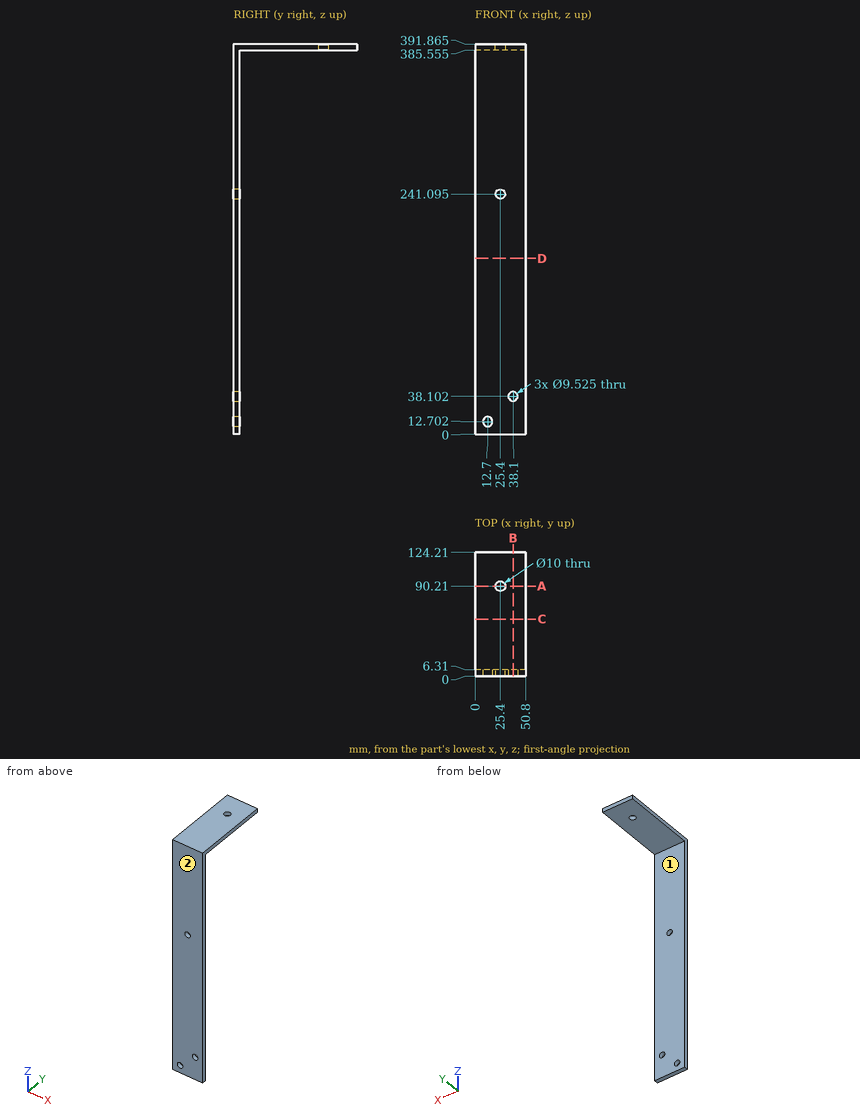
Could you check a few things on this drawing? It's one solid part, dimensions in mm from its lowest x, y, z. A direction names the side the tool comes from. Coordinates: 2 decimals unless noted, no trailing zeros. Write each loop counter-clockwise with the first axis right and the second up, starting at its lowest first coordinate (ties: lowest second). Pieces come first, ordered by that corner, then holes. Notation, with made-up numbers: M 27.25,-25.5 L 41.25,-25.5 A18 ccw 41.25,-18.5 Z; hole C 88,43.5 d4. An arc over 180 degrees is marked long. Answer as CSV lines item,"result". Start each with the question number.
Q1. Suppose I cut it at D-D, the plane z = 176.5. List the corners of the cut face in (x, y) for me, then the cut area to 3 significant figures.
Q2. For the marked faces 1 and 2, which set-ups out of +Z, -Z, +X, -X, +Y, -Y let a thin tool reach every point of the face, with its end or its side?
Q3. Suppose I cut it at A-A, the plane y = 90.21. List the corners of the cut face in (x, z) for me (3 decimals).
Q4. Suppose I cut it at B-B, the plane x = 38.1. List the corners of the cut face in (y, z) for me (1 decimal).
Q5. Suppose I cut it at C-C, the plane y = 57. List the corners of the cut face in (x, z) for me (3 decimals).
Q6. I need wall thicknesses on probe 1 along Z at (x, y) = (38.1, 2) (1 decimal); probe 2 along Z at (x, y) = (12.7, 3) (1 decimal); probe 3 along Z at (x, y) = (36, 72) (3 decimals). Which ranges of each line are inside material? Lowest first, please. Write a range as [from, to].
Q7. Will these pins go through, and if not, where does the flat tip stop? pin 1 Ø12 at (x, z) = (29, 93) entering from +Y; pin 2 Ø15 at (x, y) = (18.5, 56) entering from -Z (3 decimals).
Entries:
1,outline,"M 0,0 L 50.8,0 L 50.8,6.31 L 0,6.31 Z"
1,area,"321 mm²"
2,face 1,"-Z, +X, -X, +Y"
2,face 2,"+Z, -Z, +X, -X, -Y"
3,outline,"M 0,385.555 L 20.4,385.555 L 20.4,391.865 L 0,391.865 Z; M 30.4,385.555 L 50.8,385.555 L 50.8,391.865 L 30.4,391.865 Z"
4,outline,"M 0,0 L 6.3,0 L 6.3,33.3 L 0,33.3 Z; M 0,42.9 L 6.3,42.9 L 6.3,385.6 L 124.2,385.6 L 124.2,391.9 L 0,391.9 Z"
5,outline,"M 0,385.555 L 50.8,385.555 L 50.8,391.865 L 0,391.865 Z"
6,probe 1,"z = [0, 33.3], [42.9, 391.9]"
6,probe 2,"z = [0, 7.9], [17.5, 391.9]"
6,probe 3,"z = [385.555, 391.865]"
7,pin 1,"stops at y = 6.31"
7,pin 2,"stops at z = 385.555"
